Autodesk Inventor part; units mm, degrees
ref_plane "YZ Plane" through (0, 0, 0) normal (1, 0, 0) x (0, 1, 0)
ref_plane "XZ Plane" through (0, 0, 0) normal (0, 1, 0) x (-1, 0, 0)
ref_plane "XY Plane" through (0, 0, 0) normal (0, 0, 1) x (1, 0, 0)
sketch "Эскиз1" plane through (0, 0, 0) normal (0, 1, 0) x (-1, 0, 0)
  line L0 (0, 0) -> (0, 24.3)
  line L1 (0, 0) -> (0, -24.3)
  line L2 (-30, 24.3) -> (30, 24.3) construction
  line L3 (-30, 21.3) -> (30, 21.3)
  line L4 (30, 27.3) -> (-30, 27.3)
  arc A0 (-30, 27.3) -> (-30, 21.3) centre (-30, 24.3) ccw
  arc A1 (30, 21.3) -> (30, 27.3) centre (30, 24.3) ccw
  line L5 (-30, -24.3) -> (30, -24.3) construction
  line L6 (-30, -27.3) -> (30, -27.3)
  line L7 (30, -21.3) -> (-30, -21.3)
  arc A2 (-30, -21.3) -> (-30, -27.3) centre (-30, -24.3) ccw
  arc A3 (30, -27.3) -> (30, -21.3) centre (30, -24.3) ccw
  line L8 (-33, 24.3) -> (-33, 30.3)
  line L9 (-33, 30.3) -> (35.9111, 30.3)
  line L10 (35.9111, 30.3) -> (35.9111, -30.3)
  line L11 (35.9111, -30.3) -> (-33, -30.3)
  line L12 (-33, -30.3) -> (-33, 30.3)
  dimension "d0" = 24.3
  dimension "d1" = 24.3
  dimension "d2" = 30
  dimension "d3" = 6
  dimension "d4" = 6
  dimension "d5" = 6
  dimension "d6" = 6
extrude "Выдавливание1" add sketch "Эскиз1" along normal blind 4 contours L1 L7 A2 L12 A0 L3 L0 | L0 L3 A1 L4 A0 L8 L9 L10 L11 L12 A2 L6 A3 L7 L1
sketch "Эскиз2" plane through (0, 4, 0) normal (0, 1, 0) x (1, 0, 0)
  line L0 (33, 30.3) -> (-35.9111, 30.3)
  line L1 (33, -30.3) -> (27, -30.3)
  line L2 (27, -30.3) -> (27, 30.3)
  line L3 (27, 30.3) -> (33, 30.3)
  line L4 (33, 30.3) -> (33, -30.3)
  point P0 (0, 0)
  dimension "d9" = 6
extrude "Выдавливание2" cut sketch "Эскиз2" against normal through all
sketch "Эскиз3" plane through (0, 4, 0) normal (0, 1, 0) x (1, 0, 0)
  line L0 (27, 21.3) -> (27, -21.3)
  line L1 (27, 0) -> (27, -15)
  line L2 (27, -15) -> (27, 15)
  line L3 (27, -15) -> (-4.4812, -15)
  line L4 (-4.4812, -15) -> (-4.4812, 15)
  line L5 (-4.4812, 15) -> (27, 15)
  line L6 (27, 15) -> (27, -15)
  point P0 (0, 0)
  dimension "d12" = 15
  dimension "d13" = 30
extrude "Выдавливание3" cut sketch "Эскиз3" against normal blind 4
move faces "Перенос1" translate (-10.5, 0, 0) faces at (-4.4812, 2.6667, -5) (-21.4937, 0, 5)
sketch "Эскиз5" plane through (0, 4, 0) normal (0, 1, 0) x (1, 0, 0)
  line L0 (-35.9111, 30.3) -> (-35.9111, -30.3)
  line L1 (27, -15) -> (-14.9812, -15)
  line L2 (-35.9111, 15.0973) -> (-14.9812, 15.0973)
  line L3 (-14.9812, 15.0973) -> (-14.9812, -15)
  line L4 (-14.9812, -15) -> (-35.9111, -15)
  line L5 (-35.9111, -15) -> (-35.9111, 15.0973)
  point P0 (0, 0)
extrude "Выдавливание5" [suppressed]
sketch "Эскиз6" plane through (-35.9111, 0, 30.3) normal (0, -1, 0) x (1, 0, 0)
  line L0 (0, -45.3973) -> (20.9298, -45.3973)
  line L1 (0, -45.3973) -> (0, -42.3973)
  line L2 (0, -45.3973) -> (0, -15.3)
  line L3 (0, -15.3) -> (0, -18.3)
  line L4 (0, -42.3973) -> (15.1843, -42.3973)
  line L5 (15.1843, -42.3973) -> (15.1843, -18.3)
  line L6 (15.1843, -18.3) -> (0, -18.3)
  line L7 (0, -18.3) -> (0, -42.3973)
  point P0 (35.9111, -30.3)
  dimension "d26" = 3
  dimension "d27" = 3
extrude "Выдавливание6" [suppressed]
chamfer "Фаска1" [suppressed]
sketch "Эскиз7" plane through (0, 4, 0) normal (0, 1, 0) x (1, 0, 0)
  line L0 (-30.9111, -13.106) -> (-28.9111, -13.106)
  line L1 (-28.9111, -13.106) -> (-28.9111, -7.106)
  line L2 (-28.9111, -7.106) -> (-30.9111, -7.106)
  line L3 (-30.9111, -7.106) -> (-30.9111, -13.106)
  line L4 (-25.2291, -13.106) -> (-23.2291, -13.106)
  line L5 (-23.2291, -13.106) -> (-23.2291, -7.106)
  line L6 (-23.2291, -7.106) -> (-25.2291, -7.106)
  line L7 (-25.2291, -7.106) -> (-25.2291, -13.106)
  line L8 (0, 0) -> (-7.2083, 0)
  line L9 (-35.9111, 30.3) -> (-35.9111, -30.3)
  line L10 (-30.9111, 13.106) -> (-28.9111, 13.106)
  line L11 (-28.9111, 13.106) -> (-28.9111, 7.106)
  line L12 (-28.9111, 7.106) -> (-30.9111, 7.106)
  line L13 (-30.9111, 7.106) -> (-30.9111, 13.106)
  line L14 (-25.2291, 13.106) -> (-23.2291, 13.106)
  line L15 (-23.2291, 13.106) -> (-23.2291, 7.106)
  line L16 (-23.2291, 7.106) -> (-25.2291, 7.106)
  line L17 (-25.2291, 7.106) -> (-25.2291, 13.106)
  dimension "d33" = 2
  dimension "d34" = 6
  dimension "d35" = 2
  dimension "d36" = 5
extrude "Выдавливание7" cut sketch "Эскиз7" against normal blind 10
sketch "Эскиз8" plane through (0, 4, 0) normal (0, 1, 0) x (1, 0, 0)
  line L0 (-35.9111, 30.3) -> (-35.9111, -30.3)
  line L1 (-35.9111, 0) -> (-35.9111, -4)
  line L2 (-35.9111, -4) -> (-25.9111, -4)
  line L3 (-35.9111, -4) -> (-23.9111, -4)
  line L4 (-23.9111, -4) -> (-23.9111, 4)
  line L5 (-23.9111, 4) -> (-35.9111, 4)
  line L6 (-35.9111, 4) -> (-35.9111, -4)
  point P0 (0, 0)
  dimension "d39" = 4
  dimension "d40" = 10
  dimension "d41" = 12
  dimension "d42" = 8
extrude "Выдавливание8" cut sketch "Эскиз8" against normal blind 10
properties part number "КВ33.044.204 - Держатель ремня"
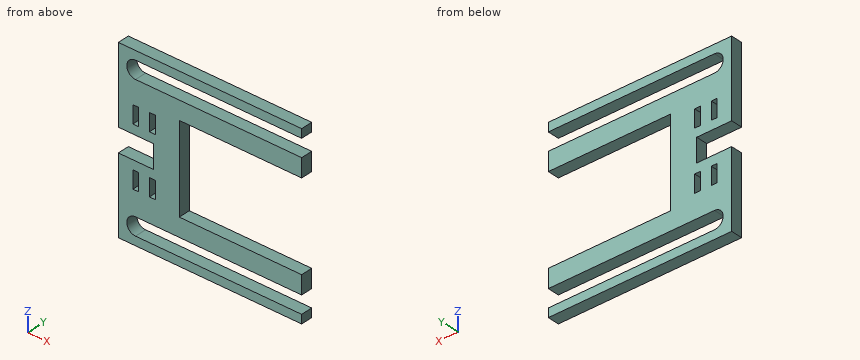
The model under review builds one solid part; all positions refer to its coordinate system, in mm. Coordinates: 2 decimals unless noted, no trailing zeros. Write each loop counter-clockwise with the first axis right and the second up, starting at its lowest first coordinate (ties: lowest second). Pieces come first, ordered by that corner, then holes. Notation, with made-up numbers: M -4,9 L 44,9 A18 ccw 44,14 Z; hole C 56.5,79 d1. An arc over 180 degrees is marked long. Put each result on its own line as item: value.
1) Wall thickness on probe 1 along Z at (x, y) = (20, 3.8); probe 2 along X at (y, z) = (2.35, 8); probe 3 along Z at (x, y) = (-17.5, 1.2): over which ranges is each line inside the solid? List them lowest first. Write a range as [from, to].
Computed:
probe 1: z = [-30.3, -27.3], [-21.3, -15], [15, 21.3], [27.3, 30.3]
probe 2: x = [-35.91, -30.91], [-28.91, -25.23], [-23.23, -14.98]
probe 3: z = [-30.3, -27.3], [-21.3, 21.3], [27.3, 30.3]
2) Add section B-B on z = 8.5. Give the boundary of the cut face in (x, y), then the cut area to 3 significant figures.
Computed:
outline: M -35.91,0 L -30.91,0 L -30.91,4 L -35.91,4 Z; M -28.91,0 L -25.23,0 L -25.23,4 L -28.91,4 Z; M -23.23,0 L -14.98,0 L -14.98,4 L -23.23,4 Z
area: 67.7 mm2
3) Clearance check with flat-ended pins moving along their axes: pin 1 Ø2 at (y, z) = (1.5, 1) entering from -X; pin 2 Ø1.5 at (y, z) = (2, -4) entering from +X. State where each tip first meets the part, or that it passes through.
Computed:
pin 1: stops at x = -23.91
pin 2: stops at x = -14.98
4) Add section D-D on z = 24.3. Give the boundary of the cut face in (x, y), then the cut area to 3 significant figures.
Computed:
outline: M -35.91,0 L -33,0 L -33,4 L -35.91,4 Z
area: 11.6 mm2
5) Add section C-C on y = 3.2. State how many separate pieces and enclosed holes the cut face has, then the cut area to 3 significant figures.
Computed:
separate pieces: 1
enclosed holes: 4
area: 1,700 mm2
6) Add section A-A on x = 8. Give the boundary of the cut face in (y, z), then the cut area to 3 significant figures.
Computed:
outline: M 0,-30.3 L 4,-30.3 L 4,-27.3 L 0,-27.3 Z; M 0,-21.3 L 4,-21.3 L 4,-15 L 0,-15 Z; M 0,15 L 4,15 L 4,21.3 L 0,21.3 Z; M 0,27.3 L 4,27.3 L 4,30.3 L 0,30.3 Z
area: 74.4 mm2
